```python
from build123d import *

# Parameters (mm, degrees)
SKETCH1_R           = 7.1
BOSS_EXTRUDE1_DEPTH = 10.5
SKETCH2_R           = 11.5
BOSS_EXTRUDE2_DEPTH = 1
SKETCH3_W           = 5
SKETCH3_H           = 3
CUT_EXTRUDE1_DEPTH  = 6


with BuildPart() as part:
    # Sketch1 → Boss-Extrude1 (new body)
    with BuildSketch(Plane(origin=(0, 0, 0), x_dir=(1, 0, 0), z_dir=(0, 1, 0))):
        Circle(SKETCH1_R)
    extrude(amount=BOSS_EXTRUDE1_DEPTH)

    # Sketch2 → Boss-Extrude2 (add)
    with BuildSketch(Plane(origin=(0, 10.5, 0), x_dir=(1, 0, 0), z_dir=(0, 1, 0))):
        Circle(SKETCH2_R)
    extrude(amount=BOSS_EXTRUDE2_DEPTH)

    # Sketch3 → Cut-Extrude1 (cut)
    with BuildSketch(Plane.XZ):
        Rectangle(SKETCH3_W, SKETCH3_H)
    extrude(amount=-CUT_EXTRUDE1_DEPTH, mode=Mode.SUBTRACT)


solid = part.part
```
CAD build for the part. Positions are in the model's coordinates, mm. A direction names the side the tool comes from. Round coordinates to 2 decimals unless told otherwise and drop trailing zeros. Write each loop counter-clockwise with the first axis right and the second up, starting at its lowest first coordinate (ties: lowest second). Pieces come first, ordered by that corner, then holes.
Item 1: Tool access for faces 4 (the flat face through (0, 3, -1.5)), 5 (the cylindrical face through (-1.5, 11, -11.4)): list every direction of +Z, -Z, +X, -X, +Y, -Y with a clear straight run to the whole face (end or side of a thin tool).
Filled in:
face 4: -Y
face 5: +Y, -Y
Item 2: Band-saw the part on C-C on y = 1.25. Write the cut outline in (x, z), then the cut area to 3 significant figures.
Filled in:
outline: circle Ø14.2 at (0, 0); hole (-2.5, -1.5) - (2.5, -1.5) - (2.5, 1.5) - (-2.5, 1.5) - close
area: 143 mm2
Item 3: Band-saw the part on A-A on x = 0. Write the cut outline in (y, z), then the cut area to 3 significant figures.
Filled in:
outline: (0, -7.1) - (10.5, -7.1) - (10.5, -11.5) - (11.5, -11.5) - (11.5, 11.5) - (10.5, 11.5) - (10.5, 7.1) - (0, 7.1) - (0, 1.5) - (6, 1.5) - (6, -1.5) - (0, -1.5) - close
area: 154 mm2
Item 4: Drop flat-ended pins along their axis: pin 1 Ø1.5 at (x, y) = (-1, 4) entering from -Z; pin 2 Ø3.5 at (y, z) = (2.5, -0.5) entering from +X; pin 3 Ø3 at (x, z) = (-9, 3) entering from -Y. Give the stop position or say it passes through.
Filled in:
pin 1: stops at z = -7.1
pin 2: stops at x = 7.1
pin 3: stops at y = 10.5
Item 5: Band-saw the part on D-D on y = 8.5. Write the cut outline in (x, z).
Filled in:
outline: circle Ø14.2 at (0, 0)
Item 6: Band-saw the part on B-B on z = 0. Write the cut outline in (x, y), then the cut area to 3 significant figures.
Filled in:
outline: (-11.5, 10.5) - (-7.1, 10.5) - (-7.1, 0) - (-2.5, 0) - (-2.5, 6) - (2.5, 6) - (2.5, 0) - (7.1, 0) - (7.1, 10.5) - (11.5, 10.5) - (11.5, 11.5) - (-11.5, 11.5) - close
area: 142 mm2
Item 7: Drill centre lines: L1, parallel to Y at x = 6.75, z = -7; L2, parallel to Z at x = -0.75, y = 9.25; L3, parallel to Z at x = 0.75, y = 11.25. Where is each one in solid material? Low to high.
Filled in:
L1: y = 10.5 to 11.5
L2: z = -7.06 to 7.06
L3: z = -11.48 to 11.48
Item 8: Mould opens along X. For faces 1 (the flat face through (0, 0, -2)), 2 (the cylindrical face through (-0.92, 5.18, -7.04)), 3 (the flat face through (0, 3, 1.5)) say: released by +X, released by -X, zero draft, split by the parting line, or undercut.
Filled in:
face 1: zero draft
face 2: split by the parting line
face 3: undercut
